Geometry: final body of the model. Coordinates: model frame, mm. A direction names the side the tool comes from. Round coordinates to 2 decimals unless told otherwise and drop trailing zeros. Loops run counter-clockwise (first coordinate to the right, second up) from the corner with the lowest first, then second, coordinate; pieces in that order, holes last. Notation, with made-up numbers: (79.5, 39) - (115.5, 39) arc R25 cw to (115.5, 58) - close; hole circle Ø7 at (12.25, 46). An arc over 180 degrees is marked (long way). Return JSON: item names as keys, results as strings. Group by question number.
1. Section A-A on z = 0. Return loops of the section in (x, y).
2. Section C-C on y = 2.5. Return loops of the section in (x, z).
3. Draft query along Z for faces 4 (the face through (45, -72, -1)), 5 (the face through (-1, -70, 50)), 6 (the face through (1, -72, 55)). Return one class per face: +Z half, -Z half, draft (parallel to the pull), parting line (faces both ways), or undercut.
4. Section B-B on x = 0. Return loops of the section in (y, z), and give its area (3 significant figures).
5. Material intervals for probe 1 along Z at (x, y) = (0, 7.5); probe 2 along Z at (x, y) = (-36.5, -41); probe 3 along X at (y, z) = (-46.5, -41), sorted ascending.
6. First-contact query: pin 1 Ø4 at (y, z) = (-51, 43.5) entering from +X; pin 2 Ø5 at (x, z) = (51.5, 6) entering from +Y; pin 3 Ø5 at (x, z) = (-33, -4.5) entering from -Y. Flat tips, straight axial feed; report the tip coordinate or a pass-through.
7. Set-up query: faces 1 (the face through (-1, -72, -45)), 2 (the face through (-15.85, 4.93, 30.474)), 3 (the face through (-1, -72, -55)). Return all of +Z, -Z, +X, -X, +Y, -Y with unobstructed straight access to the full face (end or side cutting, diameter ignored); none if empty.
8. Section D-D on z = -30.5. Count the separate pieces of the cut face and the enclosed holes in it, and give its area (3 significant figures).
Autodesk Inventor part; units mm, degrees
ref_plane "Work Plane1" through (0, -70, 0) normal (0, -1, 0) x (1, 0, 0)
ref_plane "YZ Plane" through (0, 0, 0) normal (1, 0, 0) x (0, 1, 0)
ref_plane "XZ Plane" through (0, 0, 0) normal (0, 1, 0) x (-1, 0, 0)
sketch "Sketch1" plane through (0, 0, 0) normal (0, 1, 0) x (-1, 0, 0)
  circle A0 centre (0, 0) radius 24.35
  circle A1 centre (0, 0) radius 34.35
  dimension "d0" = 48.7
  dimension "d1" = 10
extrude "Extrusion1" add sketch "Sketch1" along normal blind 10
ref_plane "Work Plane1" through (0, -70, 0) normal (0, -1, 0) x (1, 0, 0)
sketch "Sketch2" plane through (0, -70, 0) normal (0, -1, 0) x (1, 0, 0)
  circle A0 centre (0, 0) radius 34.35
  circle A1 centre (0, 0) radius 24.35
  line L0 (55, 55) -> (-55, 55)
  line L1 (-55, 55) -> (-55, -55)
  line L2 (-55, -55) -> (55, -55)
  line L3 (55, -55) -> (55, 55)
  line L4 (55, 55) -> (-55, -55) construction
  line L5 (-55, 55) -> (55, -55) construction
  line L6 (45, 45) -> (-45, 45)
  line L7 (-45, 45) -> (-45, -45)
  line L8 (-45, -45) -> (45, -45)
  line L9 (45, -45) -> (45, 45)
  line L10 (45, 45) -> (-45, -45) construction
  line L11 (-45, 45) -> (45, -45) construction
  dimension "d7" = 110
  dimension "d8" = 110
  dimension "d9" = 90
  dimension "d10" = 90
extrude "Extrusion2" add sketch "Sketch2" along normal blind 5 contours L3 L2 L1 L0
sketch "Sketch3" plane through (0, -70, 0) normal (0, 1, 0) x (1, 0, 0)
  line L0 (-55, 55) -> (55, 55)
  line L1 (45, -45) -> (45, 45)
  line L2 (55, 55) -> (45, 55)
  line L3 (45, 55) -> (45, 45)
  line L4 (45, 45) -> (55, 45)
  line L5 (55, 45) -> (55, 55)
  line L6 (-45, 45) -> (-45, -45)
  line L7 (-55, 55) -> (-45, 55)
  line L8 (-45, 55) -> (-45, 45)
  line L9 (-45, 45) -> (-55, 45)
  line L10 (-55, 45) -> (-55, 55)
  line L11 (55, -55) -> (-55, -55)
  line L12 (-55, -55) -> (-45, -55)
  line L13 (-45, -55) -> (-45, -45)
  line L14 (-45, -45) -> (-55, -45)
  line L15 (-55, -45) -> (-55, -55)
  line L16 (55, -55) -> (45, -55)
  line L17 (45, -55) -> (45, -45)
  line L18 (45, -45) -> (55, -45)
  line L19 (55, -45) -> (55, -55)
  point P0 (0, 0)
sketch "Sketch4" plane through (0, 0, 0) normal (0, -1, 0) x (1, 0, 0)
  line L0 (-55, 55) -> (-55, -55)
  line L1 (-55, -55) -> (55, -55)
  line L2 (55, -55) -> (55, 55)
  line L3 (55, 55) -> (-55, 55)
  line L4 (45, 45) -> (45, -45)
  line L5 (45, -45) -> (-45, -45)
  line L6 (-45, -45) -> (-45, 45)
  line L7 (-45, 45) -> (45, 45)
  line L8 (55, 55) -> (-55, -55)
  line L9 (-55, 55) -> (55, -55)
  line L10 (55, -55) -> (45, -55)
  line L11 (45, -55) -> (45, -45)
  line L12 (45, -45) -> (55, -45)
  line L13 (55, -45) -> (55, -55)
  line L14 (24.4112, -24.4112) -> (17.4112, -24.4112)
  line L15 (17.4112, -24.4112) -> (17.4112, -17.4112)
  line L16 (17.4112, -17.4112) -> (24.4112, -17.4112)
  line L17 (24.4112, -17.4112) -> (24.4112, -24.4112)
  line L18 (24.4112, 17.4112) -> (17.4112, 17.4112)
  line L19 (17.4112, 17.4112) -> (17.4112, 24.4112)
  line L20 (17.4112, 24.4112) -> (24.4112, 24.4112)
  line L21 (24.4112, 24.4112) -> (24.4112, 17.4112)
  line L22 (-17.2122, 17.4112) -> (-24.2122, 17.4112)
  line L23 (-24.2122, 17.4112) -> (-24.2122, 24.4112)
  line L24 (-24.2122, 24.4112) -> (-17.2122, 24.4112)
  line L25 (-17.2122, 24.4112) -> (-17.2122, 17.4112)
  line L26 (-17.4112, -24.4112) -> (-24.4112, -24.4112)
  line L27 (-24.4112, -24.4112) -> (-24.4112, -17.4112)
  line L28 (-24.4112, -17.4112) -> (-17.4112, -17.4112)
  line L29 (-17.4112, -17.4112) -> (-17.4112, -24.4112)
  point P0 (0, 0)
  dimension "d13" = 7
  dimension "d14" = 7
  dimension "d15" = 7
  dimension "d16" = 7
  dimension "d17" = 7
  dimension "d18" = 7
  dimension "d19" = 7
  dimension "d20" = 7
loft "Loft1" add profiles "Sketch4", "Sketch3" contours L27 L28 L8 | L8 L29 L26 / L0 L8 L9 L10
pattern_circular "Circular Pattern1" count 4 over 360 about axis through (0, 0, 0) along (0, 1, 0) of "Loft1"
equation "\"BendRadius\" = Thickness"
equation "\"BendReliefWidth\" = Thickness"
equation "\"BendReliefDepth\" = 0.5 * Thickness"
equation "\"CornerReliefSize\" = 4 * Thickness"
equation "\"MinimumRemnant\" = 2 * Thickness"
equation "\"TransitionRadius\" = BendRadius"
equation "\"JacobiRadiusSize\" = BendRadius"
equation "\"GapSize\" = Thickness"
properties part number "klec_1"
Taken from the geometry:
{
 "1": {"outline": "(-55, -75) - (-45, -75) - (-45, -70) - (-55, -70) - close; (-34.35, 0) - (-24.35, 0) - (-24.35, 10) - (-34.35, 10) - close; (24.35, 0) - (34.35, 0) - (34.35, 10) - (24.35, 10) - close; (45, -75) - (55, -75) - (55, -70) - (45, -70) - close"},
 "2": {"outline": "circle Ø68.7 at (0, 0); hole circle Ø48.7 at (0, 0)"},
 "3": {"face 4": "undercut", "face 5": "draft", "face 6": "+Z half"},
 "4": {"outline": "(-75, -55) - (-70, -55) - (-70, -45) - (-75, -45) - close; (-75, 45) - (-70, 45) - (-70, 55) - (-75, 55) - close; (0, -34.35) - (10, -34.35) - (10, -24.35) - (0, -24.35) - close; (0, 24.35) - (10, 24.35) - (10, 34.35) - (0, 34.35) - close", "area": "300 mm2"},
 "5": {"probe 1": "-34.35 to -24.35, 24.35 to 34.35", "probe 2": "-42.33 to -33.57, 33.57 to 42.33", "probe 3": "-44.73 to -35.74, 35.74 to 44.73"},
 "6": {"pin 1": "x = 47.57", "pin 2": "y = -70", "pin 3": "y = 0"},
 "7": {"face 1": "-Y", "face 2": "+Y", "face 3": "-Z, +X, -X, +Y, -Y"},
 "8": {"separate pieces": "5", "enclosed holes": "0", "area": "725 mm2"}
}
